Autodesk Fusion 360 part; units mm, degrees
sketch "Sketch1" plane through (0, 0, 0) normal (0, 0, 1) x (1, 0, 0)
  line L0 (0, 0) -> (30, 0)
  line L1 (30, 0) -> (30, 30)
  line L2 (30, 30) -> (0, 30)
  line L3 (0, 30) -> (0, 0)
  dimension "d10" = 30
  dimension "d11" = 30
extrude "Extrude1" add sketch "Sketch1" along normal blind 11
sketch "Sketch2" plane through (0, 0, 0) normal (1, 0, 0) x (0, 1, 0)
  line L0 (-5, 0) -> (35, 0)
  line L1 (35, 0) -> (35, 40)
  line L2 (35, 40) -> (-5, 40)
  line L3 (-5, 40) -> (-5, 0)
  dimension "d14" = 40
  dimension "d15" = 40
extrude "Extrude2" add sketch "Sketch2" against normal blind 13
hole "Hole1" at (15, 15, 11) direction (0, 0, -1) diameter 6 depth 15 tip angle 118
sketch "Sketch3" plane through (0, 0, 11) normal (0, 0, 1) x (-1, 0, 0)
  circle A0 centre (-15, -15) radius 3
  line L0 (0, -30) -> (0, 0)
  line L1 (0, 0) -> (-30, 0)
  line L2 (-30, 0) -> (-30, -30)
  line L3 (-30, -30) -> (0, -30)
  circle A1 centre (-15, -15) radius 11
  circle A2 centre (-4, -15) radius 1 construction
  circle A3 centre (-15, -26) radius 0.8867 construction
  circle A4 centre (-26, -15) radius 1 construction
  circle A5 centre (-15, -4) radius 0.9365 construction
  dimension "d23" = 22
hole "Hole2" at (4, 15, 11) at (15, 26, 11) at (26, 15, 11) at (15, 4, 11) direction (0, 0, -1) diameter 6 end through all
sketch "Sketch4" plane through (0, 0, 0) normal (1, 0, 0) x (0, 1, 0)
  line L0 (30, 11) -> (30, 0)
  line L1 (30, 0) -> (35, 0)
  line L2 (35, 0) -> (35, 40)
  line L3 (35, 40) -> (-5, 40)
  line L4 (-5, 40) -> (-5, 0)
  line L5 (-5, 0) -> (0, 0)
  line L6 (0, 0) -> (0, 11)
  line L7 (0, 11) -> (30, 11)
  line L8 (15, 40) -> (15, 11) construction
  line L9 (15, 25.5) -> (-5, 25.5) construction
  line L10 (15, 25.5) -> (35, 25.5) construction
  circle A0 centre (15, 25.5) radius 9.5525 construction
  circle A1 centre (15, 35.0525) radius 0.9475 construction
  circle A2 centre (24.5525, 25.5) radius 0.7982 construction
  circle A3 centre (15, 15.9475) radius 1.0525 construction
  circle A4 centre (5.4475, 25.5) radius 0.8032 construction
hole "Hole3" at (0, 15, 35.0525) at (0, 24.5525, 25.5) at (0, 15, 15.9475) at (0, 5.4475, 25.5) direction (-1, 0, 0) diameter 6 end through all
fillet "Fillet1" radius 3 1 edges at (0, 15, 11)
ref_plane "WorkPlane1" through (15, 15, 7) normal (0, -1, 0) x (1, 0, 0)
sketch "Sketch5" plane through (0, 15, 0) normal (0, -1, 0) x (-1, 0, 0)
equation "b1 = 30 mm"
equation "h1 = 11 mm"
equation "L1 = 30 mm"
equation "b2 = 40 mm"
equation "h2 = 13 mm"
equation "L2 = 40 mm"
equation "hole_wall = 3.4 mm"
equation "hole_motor = 3.4 mm"
equation "hole_shaft = 6 mm"
equation "d10 = b1"
equation "d11 = L1"
equation "d12 = h1"
equation "d14 = b2"
equation "d15 = L2"
equation "d16 = -h2"
equation "d19 = hole_shaft"
Verification items for the finished model (mm, model axes). A direction names the side the tool comes from. Coordinates: 2 decimals unless noted, no trailing zeros. Write each loop counter-clockwise with the first axis right and the second up, starting at its lowest first coordinate (ties: lowest second). Pieces come first, ordered by that corner, then holes. Notation, with made-up numbers: (55.5, -9.75) - (91.5, -9.75) arc R10 cw to (91.5, -1.75) - close; hole circle Ø11 at (3, 66). An arc over 180 degrees is marked (long way). Answer as a JSON object with one key per item and string values.
(1) Tool access check on faces 4 (the flat face through (-6, -5, 20)), 5 (the flat face through (15, 0, 5)), 6 (the flat face through (15, 30, 5)), 7 (the flat face through (19, 15, 11)). Record the directions out of +Z, -Z, +X, -X, +Y, -Y that give a thin tool (end or side, any length) a straight path to the whole face; none if there is none.
Report:
{"face 4": "+Z, -Z, +X, -X, -Y", "face 5": "+Z, -Z, +X, -Y", "face 6": "+Z, -Z, +X, +Y", "face 7": "+Z, +X, +Y, -Y"}
(2) Cross-section at C-C on x = 4. Record the cut outline in (y, z), plus the area to 3 significant figures.
Report:
{"outline": "(0, 0) - (12, 0) - (12, 11) - (0, 11) - close; (18, 0) - (30, 0) - (30, 11) - (18, 11) - close", "area": "264 mm^2"}
(3) Thickness scan on line 1 along X through (y, z) = (15, 6.25); line 2 along Z through (x, y) = (-2.5, 24.5); line 3 along Y through (x, z) = (-9, 25). Record the ranges inside material, lowest first.
Report:
{"line 1": "-13 to 1, 7 to 12, 18 to 23, 29 to 30", "line 2": "0 to 22.5, 28.5 to 40", "line 3": "-5 to 2.49, 8.41 to 21.59, 27.51 to 35"}
(4) Gauge pin test, flat ends, axial feed: pin 1 Ø11 at (x, z) = (12, 6) entering from +Y; pin 2 Ø5.5 at (x, y) = (15, 26) entering from +Z; pin 3 Ø7 at (y, z) = (15, 15.95) entering from +X; pin 4 Ø8 at (x, y) = (22.5, 17) entering from +Z. Record the tip position at first contact, or that the pin passes through.
Report:
{"pin 1": "y = 30", "pin 2": "through", "pin 3": "x = 0.09", "pin 4": "z = 11"}
(5) Cross-section at B-B on x = 15. Record the cut outline in (y, z), plus the area to 3 significant figures.
Report:
{"outline": "(0, 0) - (1, 0) - (1, 11) - (0, 11) - close; (7, 0) - (12, 0) - (12, 11) - (7, 11) - close; (18, 0) - (23, 0) - (23, 11) - (18, 11) - close; (29, 0) - (30, 0) - (30, 11) - (29, 11) - close", "area": "132 mm^2"}
(6) Cross-section at A-A on z = 8. Record the cut outline in (x, y).
Report:
{"outline": "(-13, -5) - (0, -5) - (0, 0) - (30, 0) - (30, 30) - (0, 30) - (0, 35) - (-13, 35) - close; hole circle Ø6 at (4, 15); hole circle Ø6 at (15, 4); hole circle Ø6 at (15, 15); hole circle Ø6 at (15, 26); hole circle Ø6 at (26, 15)"}
(7) Cross-section at D-D on y = 26. Record the cut outline in (x, z).
Report:
{"outline": "(-13, 0) - (12, 0) - (12, 11) - (3, 11) arc R3 cw to (0, 14) - (0, 22.87) - (-13, 22.87) - close; (-13, 28.13) - (0, 28.13) - (0, 40) - (-13, 40) - close; (18, 0) - (30, 0) - (30, 11) - (18, 11) - close"}
(8) Mould release check, pull along X, two halves, no side actions. Record for faces 1 (the cylindrical face through (16.8, 17.4, 5.4)), 2 (the flat face through (9, 15, 0)), 3 (the flat face through (-13, 15, 20)): pulls with the +X half, pulls with the -X half, needs draft (parallel to the pull), parting line crosses it, or undercut.
Report:
{"face 1": "undercut", "face 2": "needs draft", "face 3": "pulls with the -X half"}
